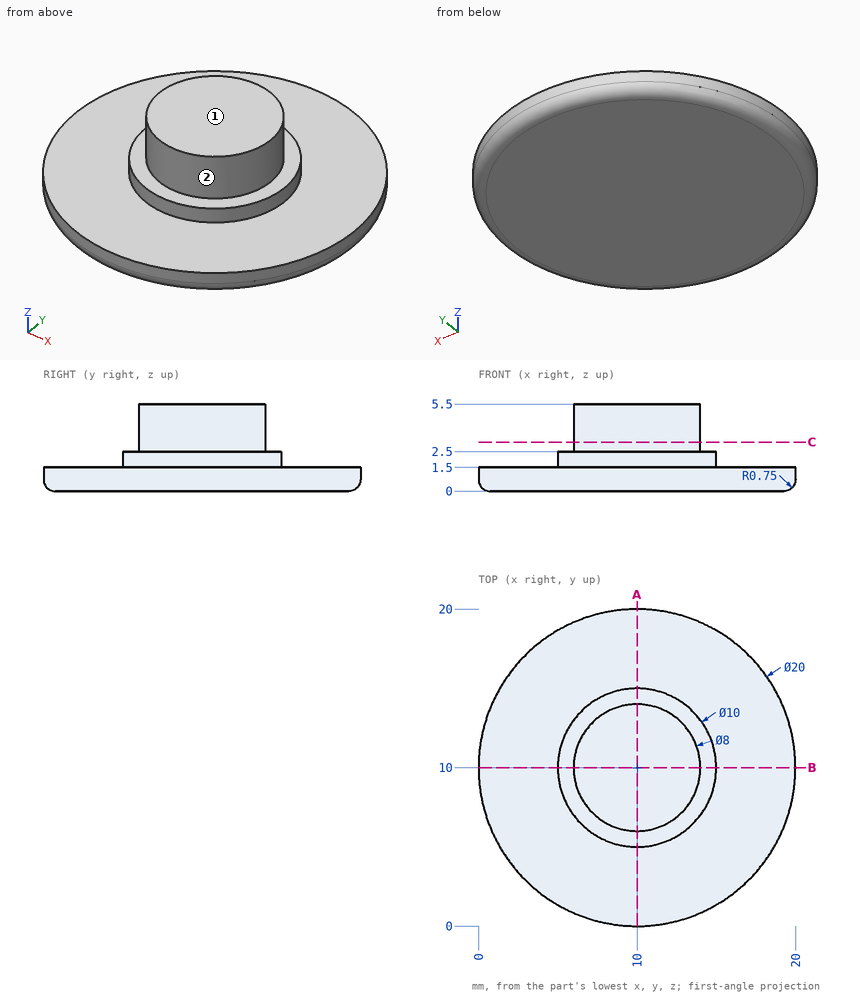
Source: three-view drawing plus pictorial views. Frame: mm from the lowest corner of the part. A direction names the side the tool comes from. Coordinates: 2 decimals unless noted, no trailing zeros. Loops run counter-clockwise (first coordinate to the right, second up) from the corner with the lowest first, then second, coordinate; pieces in that order, holes last. Notation, with made-up numbers: (75, 7) -> (125, 7) arc R24 cw to (125, 19) -> close; hole circle Ø2 at (89, 14). An arc over 180 degrees is marked (long way). One line per item, written item: value.
(1) Set-up query: the marked faces 1 and 2. Return all of +Z, -Z, +X, -X, +Y, -Y with unobstructed straight access to the full face (end or side cutting, diameter ignored); none if empty.
Answer below:
face 1: +Z, +X, -X, +Y, -Y
face 2: +Z
(2) Cut plane A-A (x = 10). Output: boundary loops of the cut face in (y, z).
Answer below:
outline: (0, 0.75) arc R0.75 ccw to (0.75, 0) -> (19.25, 0) arc R0.75 ccw to (20, 0.75) -> (20, 1.5) -> (15, 1.5) -> (15, 2.5) -> (14, 2.5) -> (14, 5.5) -> (6, 5.5) -> (6, 2.5) -> (5, 2.5) -> (5, 1.5) -> (0, 1.5) -> close
(3) Ray query, line 1 along Z through (x, y) = (14.5, 13.5); line 2 along Z through (x, y) = (6.25, 13); line 3 along X through (y, z) = (14, 2.2). Return the intervals inside material, ascending.
Answer below:
line 1: z = 0 to 1.5
line 2: z = 0 to 2.5
line 3: x = 7 to 13
(4) Pin query (flat end, axial travel): pin 1 Ø1 at (x, y) = (14, 3) entering from +Z. Return the tip coordinate at first contact, or that it passes through.
Answer below:
pin 1: stops at z = 1.5
(5) Cut plane C-C (z = 3.1). Output: boundary loops of the cut face in (x, y).
Answer below:
outline: circle Ø8 at (10, 10)
